Source: CAD feature listing. Evaluate the final solid. Frame: model axes, mm. A direction names the side the tool comes from. Round coordinates to 2 decimals unless told otherwise and drop trailing zeros. Order: outer loops, then holes, each group sorted by start corner. A loop starts at its lowest first (then second) coordinate and runs counter-clockwise, first axis right, second up. Notation, with made-up numbers: (-3.5, 1.5) - (4.5, 1.5) arc R20 ccw to (4.5, 37.5) - close; hole circle Ø3 at (-16, -25). An arc over 180 degrees is marked (long way). Return JSON: item names as keys, results as strings. Group by question number.
1) Access query for faces 4 (the flat face through (0, 0, 121.54)), 5 (the flat face through (3, 3, 59.54)), 6 (the flat face through (-16, 0, 5.08)). Directions: +Z, -Z, +X, -X, +Y, -Y. A direction counts if a zero-diameter tool reaches every point of the face in a straight line with its end or side. Return the directions, or none.
2) Mould query, pull axis X, two halves, no side actions, for faces 1 (the cylindrical face through (-0.83, -3.72, 90.11)), 2 (the flat face through (0, 0, 0)), 3 (the flat face through (0, 16, 5.08)). Classes: pulls with the +X half, pulls with the -X half, needs draft (parallel to the pull), parting line crosses it, or undercut.
3) Section A-A, the plane y = 0. Return loops of the section in (x, z).
4) Ray query, line 1 (Y direction, x = 0, z = 1.9); line 2 (Z direction, x = -7, y = -14); line 3 (Z direction, x = -4.5, y = 3.5). Return the intervals inside material, ascending. Write a range as from..to.
5) Section B-B, the plane x = -16. Return loops of the section in (y, z).
6) Contact query for flat-ended pins moving along their axis: P1, Ø1, axis at y = 4, z = 47, coming from the -X side; P2, Ø12, axis at y = -7.5, z = 46.5, coming from the +X side; P3, Ø12, axis at x = -16, y = 5.5, coming from the +Z side. Output: stop coordinate, or through.
7) Section C-C, the plane z = 42. Return loops of the section in (x, y), plus the area to 3 significant figures.
```python
from build123d import *

# Parameters (mm, degrees)
SKETCH1_R           = 30
BOSS_EXTRUDE1_DEPTH = 57
SKETCH2_R           = 12.7
BOSS_EXTRUDE2_DEPTH = 2.54
SKETCH3_R           = 3.81
BOSS_EXTRUDE3_DEPTH = 62
SKETCH4_R           = 2
CUT_EXTRUDE1_DEPTH  = 5.08


with BuildPart() as part:
    # Sketch1 → Boss-Extrude1 (new body)
    with BuildSketch(Plane.XY):
        with Locations(Location((0, 0, 0), (0, 0, 180))):
            Circle(SKETCH1_R)
    extrude(amount=BOSS_EXTRUDE1_DEPTH)

    # Sketch2 → Boss-Extrude2 (add)
    with BuildSketch(Plane.XY.offset(57)):
        Circle(SKETCH2_R)
    extrude(amount=BOSS_EXTRUDE2_DEPTH)

    # Sketch3 → Boss-Extrude3 (add)
    with BuildSketch(Plane.XY.offset(59.54)):
        Circle(SKETCH3_R)
    extrude(amount=BOSS_EXTRUDE3_DEPTH)

    # Sketch4 → Cut-Extrude1 (cut)
    with BuildSketch(Plane(origin=(0, 0, 0), x_dir=(-1, 0, 0), z_dir=(0, 0, -1))):
        with Locations((0, -16)):
            Circle(SKETCH4_R)
        with Locations((-16, 0)):
            Circle(SKETCH4_R)
        with Locations((0, 16)):
            Circle(SKETCH4_R)
        with Locations((16, 0)):
            Circle(SKETCH4_R)
    extrude(amount=-CUT_EXTRUDE1_DEPTH, mode=Mode.SUBTRACT)


solid = part.part
```
Geometry check:
{
 "1": {"face 4": "+Z, +X, -X, +Y, -Y", "face 5": "+Z", "face 6": "-Z"},
 "2": {"face 1": "parting line crosses it", "face 2": "needs draft", "face 3": "undercut"},
 "3": {"outline": "(-30, 0) - (-18, 0) - (-18, 5.08) - (-14, 5.08) - (-14, 0) - (14, 0) - (14, 5.08) - (18, 5.08) - (18, 0) - (30, 0) - (30, 57) - (12.7, 57) - (12.7, 59.54) - (3.81, 59.54) - (3.81, 121.54) - (-3.81, 121.54) - (-3.81, 59.54) - (-12.7, 59.54) - (-12.7, 57) - (-30, 57) - close"},
 "4": {"line 1": "-30..-18, -14..14, 18..30", "line 2": "0..57", "line 3": "0..59.54"},
 "5": {"outline": "(-25.38, 0) - (-2, 0) - (-2, 5.08) - (2, 5.08) - (2, 0) - (25.38, 0) - (25.38, 57) - (-25.38, 57) - close"},
 "6": {"P1": "x = -29.8", "P2": "x = 29.96", "P3": "z = 59.54"},
 "7": {"outline": "circle Ø60 at (0, 0)", "area": "2,830 mm2"}
}
